```python
from build123d import *

# Parameters (mm, degrees)
BOSS_EXTRUDE1_DEPTH = 4.5
SKETCH2_W           = 72
SKETCH2_H           = 28
CUT_EXTRUDE1_DEPTH  = 4.5
SKETCH3_W           = 95
SKETCH3_H           = 51
SKETCH3_W_2         = 90
SKETCH3_H_2         = 46
BOSS_EXTRUDE2_DEPTH = 5.1
SKETCH4_W           = 90
SKETCH4_H           = 46
CUT_EXTRUDE2_DEPTH  = 2
SKETCH6_R           = 1.5
BOSS_EXTRUDE3_DEPTH = 9.6
FILLET1_R           = 1


with BuildPart() as part:
    # Sketch1 → Boss-Extrude1 (new body)
    with BuildSketch(Plane(origin=(0, 0, 0), x_dir=(1, 0, 0), z_dir=(0, 1, 0))):
        Polygon((-14.974237314, -43.742281537), (-14.974237314, -30.742281537), (-38.474237314, -30.742281537), (-38.474237314, -43.742281537), (-44.224237314, -43.742281537), (-44.224237314, 40.257718463), (-38.474237314, 40.257718463), (-38.474237314, 27.257718463), (-14.974237314, 27.257718463), (-14.974237314, 40.257718463), (-9.224237314, 40.257718463), (-9.224237314, 23.757718463), (16.275762686, 23.757718463), (16.275762686, 40.257718463), (22.025762686, 40.257718463), (22.025762686, 27.257718463), (45.525762686, 27.257718463), (45.525762686, 40.257718463), (50.775762686, 40.257718463), (50.775762686, -43.742281537), (45.525762686, -43.742281537), (45.525762686, -30.742281537), (22.025762686, -30.742281537), (22.025762686, -43.742281537), (16.275762686, -43.742281537), (16.275762686, -27.242281537), (-9.224237314, -27.242281537), (-9.224237314, -43.742281537), align=None)
    extrude(amount=BOSS_EXTRUDE1_DEPTH)

    # Sketch2 → Cut-Extrude1 (cut)
    with BuildSketch(Plane(origin=(0, 4.5, 0), x_dir=(1, 0, 0), z_dir=(0, 1, 0))):
        with Locations((3.275762686, -1.742281537)):
            Rectangle(SKETCH2_W, SKETCH2_H)
    extrude(amount=-CUT_EXTRUDE1_DEPTH, mode=Mode.SUBTRACT)

    # Sketch3 → Boss-Extrude2 (add)
    with BuildSketch(Plane(origin=(0, 4.5, 0), x_dir=(1, 0, 0), z_dir=(0, 1, 0))):
        with Locations((3.275762686, -1.742281537)):
            Rectangle(SKETCH3_W, SKETCH3_H)
        with Locations((3.275762686, -1.742281537)):
            Rectangle(SKETCH3_W_2, SKETCH3_H_2, mode=Mode.SUBTRACT)
    extrude(amount=BOSS_EXTRUDE2_DEPTH)

    # Sketch4 → Cut-Extrude2 (cut)
    with BuildSketch(Plane(origin=(0, 4.5, 0), x_dir=(1, 0, 0), z_dir=(0, 1, 0))):
        with Locations((3.275762686, -1.742281537)):
            Rectangle(SKETCH4_W, SKETCH4_H)
    extrude(amount=-CUT_EXTRUDE2_DEPTH, mode=Mode.SUBTRACT)

    # Sketch6 → Boss-Extrude3 (add)
    # profile 1 of 6: a face of its own
    with BuildSketch(Plane(origin=(0, 9.6, 0), x_dir=(1, 0, 0), z_dir=(0, 1, 0))):
        with BuildLine():
            Line((-44.224237314, 23.757718463), (-47.224237314, 23.757718463))
            ThreePointArc((-47.224237314, 23.757718463), (-50.224237314, 20.757718463), (-47.224237314, 17.757718463))
            Line((-47.224237314, 17.757718463), (-44.224237314, 17.757718463))
            Line((-44.224237314, 17.757718463), (-44.224237314, 23.757718463))
        make_face()
        with Locations(Location((-47.224237314, 20.757718463, 0), (0, 0, 270))):
            Circle(SKETCH6_R, mode=Mode.SUBTRACT)
    # profile 2 of 6: a face of its own
    with BuildSketch(Plane(origin=(0, 9.6, 0), x_dir=(1, 0, 0), z_dir=(0, 1, 0))):
        with BuildLine():
            Line((50.775762686, 17.757718463), (53.775762686, 17.757718463))
            ThreePointArc((53.775762686, 17.757718463), (56.775762686, 20.757718463), (53.775762686, 23.757718463))
            Line((53.775762686, 23.757718463), (50.775762686, 23.757718463))
            Line((50.775762686, 23.757718463), (50.775762686, 17.757718463))
        make_face()
        with Locations(Location((53.775762686, 20.757718463, 0), (0, 0, 90))):
            Circle(SKETCH6_R, mode=Mode.SUBTRACT)
    # profile 3 of 6: a face of its own
    with BuildSketch(Plane(origin=(0, 9.6, 0), x_dir=(1, 0, 0), z_dir=(0, 1, 0))):
        with BuildLine():
            Line((50.775762686, -27.242281537), (53.775762686, -27.242281537))
            ThreePointArc((53.775762686, -27.242281537), (56.775762686, -24.242281537), (53.775762686, -21.242281537))
            Line((53.775762686, -21.242281537), (50.775762686, -21.242281537))
            Line((50.775762686, -21.242281537), (50.775762686, -27.242281537))
        make_face()
        with Locations(Location((53.775762686, -24.242281537, 0), (0, 0, 270))):
            Circle(SKETCH6_R, mode=Mode.SUBTRACT)
    # profile 4 of 6: a face of its own
    with BuildSketch(Plane(origin=(0, 9.6, 0), x_dir=(1, 0, 0), z_dir=(0, 1, 0))):
        with BuildLine():
            Line((-44.224237314, -21.242281537), (-47.224237314, -21.242281537))
            ThreePointArc((-47.224237314, -21.242281537), (-50.224237314, -24.242281537), (-47.224237314, -27.242281537))
            Line((-47.224237314, -27.242281537), (-44.224237314, -27.242281537))
            Line((-44.224237314, -27.242281537), (-44.224237314, -21.242281537))
        make_face()
        with Locations(Location((-47.224237314, -24.242281537, 0), (0, 0, 90))):
            Circle(SKETCH6_R, mode=Mode.SUBTRACT)
    # profile 5 of 6: a face of its own
    with BuildSketch(Plane(origin=(0, 9.6, 0), x_dir=(1, 0, 0), z_dir=(0, 1, 0))):
        with BuildLine():
            Line((6.275762686, -27.242281537), (6.275762686, -30.242281537))
            ThreePointArc((6.275762686, -30.242281537), (3.275762686, -33.242281537), (0.275762686, -30.242281537))
            Line((0.275762686, -30.242281537), (0.275762686, -27.242281537))
            Line((0.275762686, -27.242281537), (6.275762686, -27.242281537))
        make_face()
        with Locations(Location((3.275762686, -30.242281537, 0), (0, 0, 90))):
            Circle(SKETCH6_R, mode=Mode.SUBTRACT)
    # profile 6 of 6: a face of its own
    with BuildSketch(Plane(origin=(0, 9.6, 0), x_dir=(1, 0, 0), z_dir=(0, 1, 0))):
        with BuildLine():
            Line((0.275762686, 23.757718463), (6.275762686, 23.757718463))
            Line((6.275762686, 23.757718463), (6.275762686, 26.757718463))
            ThreePointArc((6.275762686, 26.757718463), (3.275762686, 29.757718463), (0.275762686, 26.757718463))
            Line((0.275762686, 26.757718463), (0.275762686, 23.757718463))
        make_face()
        with Locations(Location((3.275762686, 26.757718463, 0), (0, 0, 270))):
            Circle(SKETCH6_R, mode=Mode.SUBTRACT)
    extrude(amount=-BOSS_EXTRUDE3_DEPTH)

    # Fillet1
    fillet1_edges = [part.edges().sort_by_distance(p)[0] for p in [
        (-44.224237314, 2.25, -23.757718463),
        (50.775762686, 2.25, -23.757718463),
        (50.775762686, 2.25, 27.242281537),
        (-44.224237314, 2.25, 27.242281537),
        (-44.224237314, 2.25, 43.742281537),
        (-44.224237314, 2.25, -40.257718463),
        (-9.224237314, 2.25, -40.257718463),
        (-9.224237314, 2.25, -23.757718463),
        (16.275762686, 2.25, -23.757718463),
        (16.275762686, 2.25, -40.257718463),
        (50.775762686, 2.25, -40.257718463),
        (50.775762686, 2.25, 43.742281537),
        (16.275762686, 2.25, 43.742281537),
        (16.275762686, 2.25, 27.242281537),
        (-9.224237314, 2.25, 27.242281537),
        (-9.224237314, 2.25, 43.742281537),
    ]]
    fillet(fillet1_edges, radius=FILLET1_R)


solid = part.part
```
Part model, mm, in its own coordinate system. A direction names the side the tool comes from. Coordinates: 2 decimals unless noted, no trailing zeros. Order: outer loops, then holes, each group sorted by start corner. A loop starts at its lowest first (then second) coordinate and runs counter-clockwise, first axis right, second up. Notation, with made-up numbers: (30, 38.5) - (83, 38.5) arc R16 cw to (83, 58.5) - close; hole circle Ø7 at (38, 41). An arc over 180 degrees is marked (long way). Return JSON: item names as keys, results as strings. Group by question number.
Item 1: Cut at D-D (y = 8.25). State how many separate pieces and enclosed holes the cut face has, plus the area to 3 significant figures.
Item 2: Pin check, flat tips, straight feed: pin 1 (3.5 mm diameter, centred on y = 3.5, z = 39, fed in from +X); pin 2 (5 mm diameter, centred on x = -35, z = -29, fed in from +Y); pin 3 (5 mm diameter, centred on y = 2.5, z = -29, fed in from -X). Stop position of each tip, or through.
Item 3: Cut at B-B (z = 4). List the corners of the cut face in (x, y).
Item 4: Which spindle directions (+Z, -Z, +X, -X, +Y, -Y) get a long thin tool onto all of the face, cutting with end or side? Do faces 1 (the face through (24, 6, -23.758)), 2 (the face through (3, 1, 15.742)), 3 (the face through (34, 4.5, 30)). Say none if no direction does.
Item 5: Cut at C-C (z = 35.5). List the corners of the cut face in (x, y).
Item 6: Pull direction Z, two halves, no side cores. Call faces 4 (the face through (24, 6, 27.242)), 5 (the face through (-18, 6, -23.758)), 6 (the face through (48.276, 6, 2)), 7 (the face through (52, 5, -17.758)): pulls with the +Z half, pulls with the -Z half, needs draft (parallel to the pull), parting line crosses it, or undercut.
Item 7: Cut at A-A (x = -17). List the corners of the cut face in (y, z).
Item 8: Drill centre lines: probe 1 along X at (y, z) = (0.75, 30); probe 2 along X at (y, z) = (2.75, -33); probe 3 along Z at (x, y) = (8, 6). Where is each one in solid material? Low to high. Write a range as from..to.
Check values:
{
 "1": {"separate pieces": "1", "enclosed holes": "7", "area": "855 mm2"},
 "2": {"pin 1": "stops at x = 50.78", "pin 2": "stops at y = 4.5", "pin 3": "stops at x = -44.22"},
 "3": {"outline": "(-44.22, 0) - (-32.72, 0) - (-32.72, 2.5) - (-41.72, 2.5) - (-41.72, 9.6) - (-44.22, 9.6) - close; (39.28, 0) - (50.78, 0) - (50.78, 9.6) - (48.28, 9.6) - (48.28, 2.5) - (39.28, 2.5) - close"},
 "4": {"face 1": "-Z, +Y", "face 2": "+Y, -Y", "face 3": "+Z, +X, +Y"},
 "5": {"outline": "(-44.22, 0) - (-38.47, 0) - (-38.47, 4.5) - (-44.22, 4.5) - close; (-14.97, 0) - (-9.22, 0) - (-9.22, 4.5) - (-14.97, 4.5) - close; (16.28, 0) - (22.03, 0) - (22.03, 4.5) - (16.28, 4.5) - close; (45.53, 0) - (50.78, 0) - (50.78, 4.5) - (45.53, 4.5) - close"},
 "6": {"face 4": "pulls with the +Z half", "face 5": "pulls with the -Z half", "face 6": "undercut", "face 7": "undercut"},
 "7": {"outline": "(0, -27.26) - (4.5, -27.26) - (4.5, -23.76) - (9.6, -23.76) - (9.6, -21.26) - (2.5, -21.26) - (2.5, -12.26) - (0, -12.26) - close; (0, 15.74) - (2.5, 15.74) - (2.5, 24.74) - (9.6, 24.74) - (9.6, 27.24) - (4.5, 27.24) - (4.5, 30.74) - (0, 30.74) - close"},
 "8": {"probe 1": "x = -44.22..-9.22, 0.28..1.8, 4.76..6.28, 16.28..50.78", "probe 2": "x = -44.22..-38.47, -14.97..-9.22, 16.28..22.03, 45.53..50.78", "probe 3": "z = -23.76..-21.26, 24.74..27.24"}
}
